from build123d import *

# Parameters (mm, degrees)
SKETCH1_W            = 165.1
SKETCH1_H            = 95.25
BOSS_EXTRUDE1_DEPTH  = 6.35
CUT_EXTRUDE1_DEPTH   = 96.514216874
MIRROR2_COPY_1_DEPTH = 96.514216874


with BuildPart() as part:
    # Sketch1 → Boss-Extrude1 (new body)
    with BuildSketch(Plane(origin=(0, 0, 0), x_dir=(1, 0, 0), z_dir=(0, 1, 0))):
        Rectangle(SKETCH1_W, SKETCH1_H)
    extrude(amount=BOSS_EXTRUDE1_DEPTH)

    # Sketch2 → Cut-Extrude1 (cut, through all)
    with BuildSketch(Plane(origin=(0, 6.35, 0), x_dir=(1, 0, 0), z_dir=(0, 1, 0))):
        Polygon((82.55, -21.9075), (82.55, -25.7175), (79.1845, -25.7175), (79.1845, -27.8765), (76.3905, -27.8765), (76.3905, -25.7175), (73.025, -25.7175), (73.025, -21.9075), (76.3905, -21.9075), (76.3905, -19.7485), (79.1845, -19.7485), (79.1845, -21.9075), align=None)
    cut_extrude1 = extrude(amount=-CUT_EXTRUDE1_DEPTH, mode=Mode.SUBTRACT)

    # Mirror1: Cut-Extrude1 across plane
    add(cut_extrude1.mirror(Plane.XY), mode=Mode.SUBTRACT)

    # Mirror2: Cut-Extrude1 across plane
    add(cut_extrude1.mirror(Plane(origin=(0, 0, 0), x_dir=(0, 0, 1), z_dir=(1, 0, 0))), mode=Mode.SUBTRACT)

    # Mirror2 copy 1 sketch → Mirror2 copy 1 (cut, through all)
    with BuildSketch(Plane(origin=(0, 6.35, 0), x_dir=(-1, 0, 0), z_dir=(0, 1, 0))):
        Polygon((82.55, -21.9075), (82.55, -25.7175), (79.1845, -25.7175), (79.1845, -27.8765), (76.3905, -27.8765), (76.3905, -25.7175), (73.025, -25.7175), (73.025, -21.9075), (76.3905, -21.9075), (76.3905, -19.7485), (79.1845, -19.7485), (79.1845, -21.9075), align=None)
    extrude(amount=-MIRROR2_COPY_1_DEPTH, mode=Mode.SUBTRACT)


solid = part.part
Source: CAD feature listing. Evaluate the final solid. Frame: model axes, mm. A direction names the side the tool comes from. Give positions to 0.01 mm unless a question says otherwise; leave off trailing zeros. Write each loop counter-clockwise with the first axis right and the second up, starting at its lowest first coordinate (ties: lowest second). Pieces come first, ordered by that corner, then holes. Notation, with made-up numbers: M 66,33.5 L 97,33.5 A24 ccw 97,44.5 Z; hole C 84.5,86 d11. An arc over 180 degrees is marked long. Answer as a JSON object with one key per item and string values.
Q1. Cut plane A-A, the plane z = 24. Return the cut outline in (x, y) (3 decimals), then the cut area to 3 significant figures.
Geometry check:
{"outline": "M -73.025,0 L 73.025,0 L 73.025,6.35 L -73.025,6.35 Z", "area": "927 mm^2"}
Q2. Contact query for a flat-ended pin moving along its axis: P1, Ø1.1, axis at y = 2, z = -23, coming from the -X side (3 decimals). Output: stop coordinate, or through.
Geometry check:
{"P1": "stops at x = -73.025"}
Q3. Mould query, pull axis Z, two halves, no side actions, for faces 4 (the face through (75, 3, 25.718)), 5 (the face through (-1, 3, 47.625)), 6 (the face through (82.55, 3, -37)). Classes: +Z half, -Z half, draft (parallel to the pull), parting line (faces both ways), or undercut.
Geometry check:
{"face 4": "undercut", "face 5": "+Z half", "face 6": "draft"}
Q4. Ray query, line 1 along X through (y, z) = (1, -26); line 2 along Z through (x, y) = (-74, 5.25) (1 decimal). Return the intervals inside material, ascending.
Geometry check:
{"line 1": "x = -82.55 to -79.18, -76.39 to 76.39, 79.18 to 82.55", "line 2": "z = -47.6 to -25.7, -21.9 to 21.9, 25.7 to 47.6"}
Q5. Access query for faces 1 (the face through (73.025, 3, -24)), 2 (the face through (-82.55, 3, 37)), 3 (the face through (-75, 3, -21.908)). Directions: +Z, -Z, +X, -X, +Y, -Y. A direction counts if a zero-diameter tool reaches every point of the face in a straight line with its end or side. Return the directions, or none.
Geometry check:
{"face 1": "+X, +Y, -Y", "face 2": "+Z, -Z, -X, +Y, -Y", "face 3": "-X, +Y, -Y"}
